```python
from build123d import *

# Parameters (mm, degrees)
SKETCH1_W            = 609.6
SKETCH1_H            = 914.4
OUTERBODIE_DEPTH     = 152.4
SHELL1_T             = -8.89
SKETCH3_W            = 457.2
SKETCH3_H            = 127
WIRE_DUCT_DEPTH      = 8.89
SKETCH2_W            = 457.2
SKETCH2_H            = 457.2
DISPLAY_CUTOUT_DEPTH = 8.89
SKETCH5_W            = 88.9
SKETCH5_H            = 38.1
SKETCH5_W_2          = 31.75
GAME_DISPLAY_DEPTH   = 8.89


with BuildPart() as part:
    # Sketch1 → OuterBodie (new body)
    with BuildSketch(Plane(origin=(0, 0, 0), x_dir=(0, 0, -1), z_dir=(1, 0, 0))):
        with Locations((0, 457.2)):
            Rectangle(SKETCH1_W, SKETCH1_H)
    extrude(amount=-OUTERBODIE_DEPTH)

    # Shell1
    shell1_openings = [part.faces().sort_by_distance(p)[0] for p in [
        (-76.2, 457.2, -304.8),
    ]]
    offset(amount=SHELL1_T, openings=shell1_openings, kind=Kind.INTERSECTION)

    # Sketch3 → Wire duct (cut)
    with BuildSketch(Plane(origin=(0, 0, 0), x_dir=(0, 0, -1), z_dir=(1, 0, 0))):
        with Locations((0, 127)):
            Rectangle(SKETCH3_W, SKETCH3_H)
    extrude(amount=-WIRE_DUCT_DEPTH, mode=Mode.SUBTRACT)

    # Sketch2 → Display cutout (cut)
    with BuildSketch(Plane(origin=(0, 0, 0), x_dir=(0, 0, -1), z_dir=(1, 0, 0))):
        with Locations((0, 584.2)):
            Rectangle(SKETCH2_W, SKETCH2_H)
    extrude(amount=-DISPLAY_CUTOUT_DEPTH, mode=Mode.SUBTRACT)

    # Sketch5 → Game Display (cut)
    with BuildSketch(Plane(origin=(0, 0, 0), x_dir=(0, 0, -1), z_dir=(1, 0, 0))):
        with Locations((-209.55, 857.25)):
            Rectangle(SKETCH5_W, SKETCH5_H)
        with Locations((-82.55, 857.25)):
            Rectangle(SKETCH5_W, SKETCH5_H)
        with Locations((44.45, 857.25)):
            Rectangle(SKETCH5_W, SKETCH5_H)
        with Locations((160.026262688, 857.25)):
            Rectangle(SKETCH5_W_2, SKETCH5_H)
    extrude(amount=-GAME_DISPLAY_DEPTH, mode=Mode.SUBTRACT)


solid = part.part
```
Build history of the part. All positions in model axes, mm. A direction names the side the tool comes from. Coordinates: 2 decimals unless noted, no trailing zeros. Order: outer loops, then holes, each group sorted by start corner. A loop starts at its lowest first (then second) coordinate and runs counter-clockwise, first axis right, second up. Notation, with made-up numbers: M -32,79.5 L -25,79.5 A30 cw -25,113.5 Z; hole C -16,47 d4. An arc over 180 degrees is marked long. One line per question, with ' | ' between items. Start each with the question number.
1. Cut at D-D (y = 221). Write the cut outline in (x, z).
2. Cut at A-A (z = 52). Write the cut outline in (x, y), plus the area to 3 significant figures.
3. Cut at C-C (x = -115). Write the cut outline in (y, z), plus the area to 3 significant figures.
4. Wall check: line 1 along X through (y, z) = (413, -241.5); line 2 along Y through (x, z) = (-93.5, 191); line 3 along Z through (x, y) = (-141.5, 361.5). Give the ranges that are in metal, low to high. Write a range as [from, to].
5. Cut at B-B (y = 472). Write the cut outline in (x, z).
6. Mould opens along X. For faces 1 (the face through (-75, 451, 295.91)), 2 (the face through (-8, 455, -304.8)), 3 (the face through (0, 260, 4)) say: +X half, -X half, draft (parallel to the pull), parting line (faces both ways), or undercut.
7. Tool access for faces 4 (the face through (-75, 8.89, 0)), 5 (the face through (-75, 451, 304.8)): list every direction of +Z, -Z, +X, -X, +Y, -Y with a clear straight run to the whole face (end or side of a thin tool).
8. Flat gauge pins, fed straight in: P1, Ø2, axis at x = -97, y = 249, coming from the -Z side; P2, Ø12, axis at y = 669.5, z = 75.5, coming from the +X side. Where does each tip first touch, or does it go through?
The answers:
1) outline: M -152.4,-304.8 L -143.51,-304.8 L -143.51,295.91 L -8.89,295.91 L -8.89,-304.8 L 0,-304.8 L 0,304.8 L -152.4,304.8 Z
2) outline: M -152.4,0 L 0,0 L 0,63.5 L -8.89,63.5 L -8.89,8.89 L -143.51,8.89 L -143.51,905.51 L -8.89,905.51 L -8.89,876.3 L 0,876.3 L 0,914.4 L -152.4,914.4 Z; M -8.89,190.5 L 0,190.5 L 0,355.6 L -8.89,355.6 Z; M -8.89,812.8 L 0,812.8 L 0,838.2 L -8.89,838.2 Z | area: 13,100 mm2
3) outline: M 0,-304.8 L 8.89,-304.8 L 8.89,295.91 L 905.51,295.91 L 905.51,-304.8 L 914.4,-304.8 L 914.4,304.8 L 0,304.8 Z | area: 18,800 mm2
4) line 1: x = [-152.4, -143.51], [-8.89, 0] | line 2: y = [0, 8.89], [905.51, 914.4] | line 3: z = [295.91, 304.8]
5) outline: M -152.4,-304.8 L -143.51,-304.8 L -143.51,295.91 L -8.89,295.91 L -8.89,228.6 L 0,228.6 L 0,304.8 L -152.4,304.8 Z; M -8.89,-304.8 L 0,-304.8 L 0,-228.6 L -8.89,-228.6 Z
6) face 1: undercut | face 2: draft | face 3: +X half
7) face 4: -Z | face 5: +Z, +X, -X, +Y, -Y
8) P1: stops at z = 295.91 | P2: stops at x = -143.51
